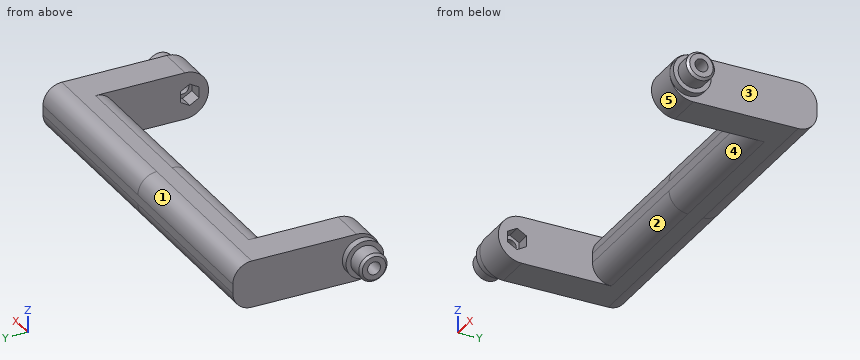
from build123d import *

# Parameters (mm, degrees)
CONNECTOR_MOUNTING_CHAMFER_SIZE              = 1
HANDLE_BODY_DEPTH                            = 10
LOWER_HANDLE_FILLET_R                        = 10
UPPER_HANDLE_FILLET_R                        = 8
MOUNTING_SCREW_HOLE_D                        = 5.5
NUT_CUTOUT_DEPTH                             = 6
LOWER_HANDLE_FILLET_OF_HANDLE_MIRROR_R       = 10
UPPER_HANDLE_FILLET_OF_HANDLE_MIRROR_R       = 8
CONNECTOR_MOUNTING_CHAMFER_OF_CONNECTOR_SIZE = 1


with BuildPart() as part:
    # Sketch1 → connector_body (revolve)
    with BuildSketch(Plane.XY, mode=Mode.PRIVATE) as connector_body_sk:
        Polygon((0, 0), (0, 8), (3, 8), (3, 6), (10.5, 6), (10.5, 0), align=None)
    connector_body = revolve(connector_body_sk.sketch.rotate(Axis((0, 0, 0), (1, 0, 0)), 90), axis=Axis((0, 0, 0), (1, 0, 0)))

    # connector_mounting_chamfer
    connector_mounting_chamfer_edges = [part.edges().sort_by_distance(p)[0] for p in [
        (10.5, 0, -6),
    ]]
    chamfer(connector_mounting_chamfer_edges, length=CONNECTOR_MOUNTING_CHAMFER_SIZE)

    # Sketch2 → handle_body (add, symmetric)
    with BuildSketch(Plane.XY):
        Polygon((0, -8), (0, 54.5), (-77.5, 54.5), (-77.5, 32), (-15, 32), (-15, -8), align=None)
    handle_body = extrude(amount=HANDLE_BODY_DEPTH, both=True)

    # lower_handle_fillet
    # the kernel refuses this fillet: 10 mm, written as the material it takes off along each edge
    with BuildSketch(Plane(origin=(-40, -8, -10), x_dir=(0, 0, 1), z_dir=(1, 0, 0))) as lower_handle_fillet_piece_1:
        with BuildLine():
            CenterArc((LOWER_HANDLE_FILLET_R, -LOWER_HANDLE_FILLET_R), LOWER_HANDLE_FILLET_R, 90, 90)
            Line((0, -LOWER_HANDLE_FILLET_R), (0, 0))
            Line((0, 0), (LOWER_HANDLE_FILLET_R, 0))
        make_face()
    extrude(amount=65, mode=Mode.SUBTRACT)
    with BuildSketch(Plane(origin=(-40, -8, 10), x_dir=(0, 0, -1), z_dir=(1, 0, 0))) as lower_handle_fillet_piece_2:
        with BuildLine():
            CenterArc((LOWER_HANDLE_FILLET_R, LOWER_HANDLE_FILLET_R), LOWER_HANDLE_FILLET_R, 180, 90)
            Line((0, LOWER_HANDLE_FILLET_R), (0, 0))
            Line((0, 0), (LOWER_HANDLE_FILLET_R, 0))
        make_face()
    extrude(amount=65, mode=Mode.SUBTRACT)

    # upper_handle_fillet
    upper_handle_fillet_edges = [part.edges().sort_by_distance(p)[0] for p in [
        (-46.25, 32, -10),
        (-38.75, 54.5, -10),
        (-38.75, 54.5, 10),
        (-46.25, 32, 10),
    ]]
    fillet(upper_handle_fillet_edges, radius=UPPER_HANDLE_FILLET_R)

    # mounting_screw_hole (through all)
    with Locations(Plane(origin=(10.5, 0, 0), x_dir=(0, 0, -1), z_dir=(1, 0, 0))):
        with Locations((0, 0)):
            mounting_screw_hole = Hole(MOUNTING_SCREW_HOLE_D / 2)

    # Sketch6 → nut_cutout (cut)
    with BuildSketch(Plane.ZY.offset(15)):
        Polygon((4.618802154, 0), (2.309401077, 4), (-2.309401077, 4), (-4.618802154, 0), (-2.309401077, -4), (2.309401077, -4), align=None)
    nut_cutout = extrude(amount=-NUT_CUTOUT_DEPTH, mode=Mode.SUBTRACT)

    # handle_mirror: handle_body across plane
    add(handle_body.mirror(Plane(origin=(-77.5, 0, 0), x_dir=(0, 0, 1), z_dir=(1, 0, 0))))

    # lower_handle_fillet of handle_mirror
    # the kernel refuses this fillet: 10 mm, written as the material it takes off along each edge
    with BuildSketch(Plane(origin=(-115, -8, -10), x_dir=(0, 1, 0), z_dir=(-1, 0, 0))) as lower_handle_fillet_of_handle_mirror_piece_1:
        with BuildLine():
            CenterArc((LOWER_HANDLE_FILLET_OF_HANDLE_MIRROR_R, -LOWER_HANDLE_FILLET_OF_HANDLE_MIRROR_R), LOWER_HANDLE_FILLET_OF_HANDLE_MIRROR_R, 90, 90)
            Line((0, -LOWER_HANDLE_FILLET_OF_HANDLE_MIRROR_R), (0, 0))
            Line((0, 0), (LOWER_HANDLE_FILLET_OF_HANDLE_MIRROR_R, 0))
        make_face()
    extrude(amount=65, mode=Mode.SUBTRACT)
    with BuildSketch(Plane(origin=(-115, -8, 10), x_dir=(0, 1, 0), z_dir=(-1, 0, 0))) as lower_handle_fillet_of_handle_mirror_piece_2:
        with BuildLine():
            CenterArc((LOWER_HANDLE_FILLET_OF_HANDLE_MIRROR_R, LOWER_HANDLE_FILLET_OF_HANDLE_MIRROR_R), LOWER_HANDLE_FILLET_OF_HANDLE_MIRROR_R, 180, 90)
            Line((0, LOWER_HANDLE_FILLET_OF_HANDLE_MIRROR_R), (0, 0))
            Line((0, 0), (LOWER_HANDLE_FILLET_OF_HANDLE_MIRROR_R, 0))
        make_face()
    extrude(amount=65, mode=Mode.SUBTRACT)

    # upper_handle_fillet of handle_mirror
    upper_handle_fillet_of_handle_mirror_edges = [part.edges().sort_by_distance(p)[0] for p in [
        (-108.75, 32, -10),
        (-116.25, 54.5, -10),
        (-116.25, 54.5, 10),
        (-108.75, 32, 10),
    ]]
    fillet(upper_handle_fillet_of_handle_mirror_edges, radius=UPPER_HANDLE_FILLET_OF_HANDLE_MIRROR_R)

    # connector_mirror: connector_body, mounting_screw_hole, nut_cutout across plane
    add(connector_body.mirror(Plane(origin=(-77.5, 0, 0), x_dir=(0, 0, 1), z_dir=(1, 0, 0))))
    add(mounting_screw_hole.mirror(Plane(origin=(-77.5, 0, 0), x_dir=(0, 0, 1), z_dir=(1, 0, 0))), mode=Mode.SUBTRACT)
    add(nut_cutout.mirror(Plane(origin=(-77.5, 0, 0), x_dir=(0, 0, 1), z_dir=(1, 0, 0))), mode=Mode.SUBTRACT)

    # connector_mounting_chamfer of connector
    connector_mounting_chamfer_of_connector_edges = [part.edges().sort_by_distance(p)[0] for p in [
        (-165.5, 0, -6),
    ]]
    chamfer(connector_mounting_chamfer_of_connector_edges, length=CONNECTOR_MOUNTING_CHAMFER_OF_CONNECTOR_SIZE)


solid = part.part
Source: CAD feature listing. Evaluate the final solid. Frame: model axes, mm. Face numbers are marked on the shaded views. A direction names the side the tool comes from. Round coordinates to 2 decimals unless told otherwise and drop trailing zeros. Loops run counter-clockwise (first coordinate to the right, second up) from the corner with the lowest first, then second, coordinate; pieces in that order, holes last. Notation, with made-up numbers: (43, -34.5) - (47, -34.5) arc R21 cw to (47, -24.5) - close; hole circle Ø3 at (30.5, 33.5). An arc over 180 degrees is marked (long way). Write item = value, one per line. Start each with the question number.
Item 1: Material intervals for line 1 (Y direction, x = 0.5, z = 0); line 2 (X direction, y = 2, z = 8.75); line 3 (Y direction, x = -3.5, z = 0), sorted ascending.
Item 2: Reachability of the marked faces 4 and 5 from +Z, -Z, +X, -X, +Y, -Y: full face, straight path, thin tool, end or side. Return the list, or none.
Item 3: Section query B-B on x = -53. Output: boundary loops of the cut face in (y, z), plus the area to 3 significant figures.
Item 4: Section query A-A on y = 20. Output: boundary loops of the cut face in (x, z), plus the area to 3 significant figures.
Item 5: First-contact query: pin 1 Ø6 at (y, z) = (28, 7.5) entering from -X; pin 2 Ø3 at (x, z) = (-72.5, 0.5) entering from -Y; pin 3 Ø6.5 at (y, z) = (48.5, -5) entering from +X; pin 4 Ø2.5 at (y, z) = (-0.5, 0) entering from +X. Flat tips, straight axial feed; report the tip coordinate or a pass-through.
Item 6: Mould query, pull axis X, two halves, no side actions, for the marked faces 1, 2 and 3. Classes: released by +X, released by -X, zero draft, split by the parting line, or undercut.
Results list:
q1.line_1 = -8 to -2.75, 2.75 to 8
q1.line_2 = -155 to -140, -15 to 0
q1.line_3 = -8 to -2.75, 2.75 to 54.5
q2.face_4 = -Z, -Y
q2.face_5 = +X, -X, -Y
q3.outline = (32, -2) arc R8 ccw to (40, -10) - (46.5, -10) arc R8 ccw to (54.5, -2) - (54.5, 2) arc R8 ccw to (46.5, 10) - (40, 10) arc R8 ccw to (32, 2) - close
q3.area = 395 mm²
q4.outline = (-155, -10) - (-140, -10) - (-140, 10) - (-155, 10) - close; (-15, -10) - (0, -10) - (0, 10) - (-15, 10) - close
q4.area = 600 mm²
q5.pin_1 = -155
q5.pin_2 = 32
q5.pin_3 = 0
q5.pin_4 = through
q6.face_1 = zero draft
q6.face_2 = undercut
q6.face_3 = released by +X
